Here's how the part is built. I have some questions about the finished solid (model axes, mm). A direction names the side the tool comes from. Give positions to 0.01 mm unless a question says otherwise; leave off trailing zeros. Order: outer loops, then holes, each group sorted by start corner. A loop starts at its lowest first (then second) coordinate and runs counter-clockwise, first axis right, second up. Notation, with made-up numbers: M 1,-17.75 L 49,-17.75 A14 ccw 49,1.25 Z; hole C 26,67 d5. An arc over 180 degrees is marked long. One line per item, written item: value. Start each with the question number.
from build123d import *

# Parameters (mm, degrees)
F0_R     = 31.75
F1_DEPTH = 12.7


with BuildPart() as f1:
    # F0 (on Front) → F1 (new body)
    with BuildSketch(Plane.XZ):
        with Locations((0, -6.35)):
            Circle(F0_R)
        Polygon((-3.666174, -6.35), (-7.332348, 0), (-3.666174, 6.35), (3.666174, 6.35), (7.332348, 0), (3.666174, -6.35), align=None, mode=Mode.SUBTRACT)
    extrude(amount=F1_DEPTH)


solid = f1.part
Item 1: I want a section at D-D on z = 17. Write out the boundary of the cut face in (x, y), plus the area to 3 significant figures.
Item 2: Please list where these lines run through material, in increasing order: probe 1 along X at (y, z) = (-7.5, 3); probe 2 along Z at (x, y) = (-4, -9.75); probe 3 along X at (y, z) = (-6.5, -11.5). Write a range as [from, to].
Item 3: I want a section at C-C on z = 3. Write out the boundary of the cut face in (x, y), plus the area to 3 significant figures.
Item 4: I want a section at B-B on x = 0. Write out the boundary of the cut face in (y, z), plus the area to 3 significant figures.
Item 5: I want a section at A-A on y = -4.5. Write out the boundary of the cut face in (x, z), plus the area to 3 significant figures.
Item 6: For faces 5 (the face through (0, -6, -6.35)), 6 (the face through (0, 0, -13)), which set-ups out of +Z, -Z, +X, -X, +Y, -Y let a thin tool reach every point of the face, with its end or its side?
Item 7: Will these pins go through, and if not, where does the flat tip stop? P1, Ø6, axis at x = 0, y = -6, coming from the +Z side; P2, Ø3, axis at x = 17, y = -9.5, coming from the -Z side; P3, Ø4, axis at x = -24, y = -6, coming from the +Z side.
Item 8: We'd pull the mould along Z, two halves only. Please class faces 1 (the face through (0, -6, 6.35)), 2 (the face through (0, -12.7, -13)), 3 (the face through (30.284, -6.261, 3.187)), 4 (the face through (5.474, -6.261, 3.219)): +Z half, -Z half, draft (parallel to the pull), parting line (faces both ways), or undercut.
Answer below:
1. outline: M -21.51,-12.7 L 21.51,-12.7 L 21.51,0 L -21.51,0 Z
1. area: 546 mm²
2. probe 1: x = [-30.34, -5.6], [5.6, 30.34]
2. probe 2: z = [-37.85, -5.77], [5.77, 25.15]
2. probe 3: x = [-31.33, 31.33]
3. outline: M -30.34,-12.7 L -5.6,-12.7 L -5.6,0 L -30.34,0 Z; M 5.6,-12.7 L 30.34,-12.7 L 30.34,0 L 5.6,0 Z
3. area: 628 mm²
4. outline: M -12.7,-38.1 L 0,-38.1 L 0,-6.35 L -12.7,-6.35 Z; M -12.7,6.35 L 0,6.35 L 0,25.4 L -12.7,25.4 Z
4. area: 645 mm²
5. outline: C 0,-6.35 d63.5; hole M -7.33,0 L -3.67,-6.35 L 3.67,-6.35 L 7.33,0 L 3.67,6.35 L -3.67,6.35 Z
5. area: 3,030 mm²
6. face 5: +Y, -Y
6. face 6: +Z, -Z, +X, -X, +Y
7. P1: stops at z = 25.4
7. P2: stops at z = -34.06
7. P3: stops at z = 16.54
8. face 1: undercut
8. face 2: draft
8. face 3: parting line
8. face 4: undercut
